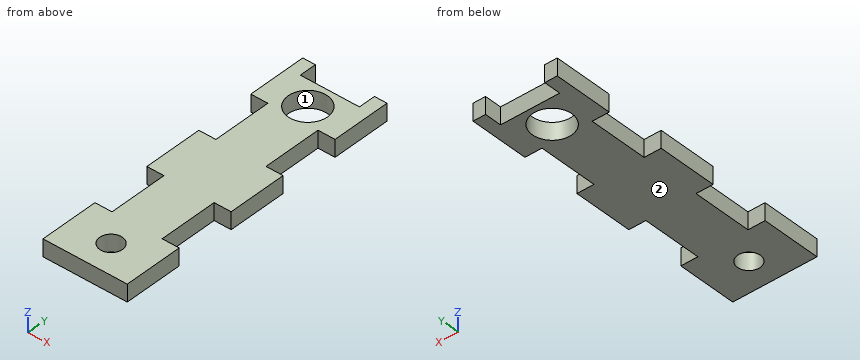
from build123d import *

# Parameters (mm, degrees)
SKETCH1_R               = 11
BOSS_EXTRUDE1_DEPTH     = 9.525
SKETCH3_R               = 6.35
CUT_EXTRUDE1_DEPTH      = 1
CUT_EXTRUDE1_DEPTH_BACK = 10.525


with BuildPart() as part:
    # Sketch1 → Boss-Extrude1 (new body)
    with BuildSketch(Plane.XY):
        Polygon((0, 0), (0, -33.02), (9.525, -33.02), (9.525, -66.04), (0, -66.04), (0, -99.06), (9.525, -99.06), (9.525, -132.08), (0, -132.08), (0, -165.1), (47.05, -165.1), (47.05, -132.08), (37.525, -132.08), (37.525, -99.06), (47.05, -99.06), (47.05, -66.04), (37.525, -66.04), (37.525, -33.02), (47.05, -33.02), (47.05, 0), (40.03499994, 0), (40.03499994, -9.525), (7.01499994, -9.525), (7.01499994, 0), align=None)
        with Locations((23.525, -23.525)):
            Circle(SKETCH1_R, mode=Mode.SUBTRACT)
    extrude(amount=BOSS_EXTRUDE1_DEPTH)

    # Sketch3 → Cut-Extrude1 (cut, two sides)
    with BuildSketch(Plane(origin=(0, 0, 0), x_dir=(-1, 0, 0), z_dir=(0, 0, -1))) as cut_extrude1_sk:
        with Locations((-23.525, -148.59)):
            Circle(SKETCH3_R)
    extrude(amount=CUT_EXTRUDE1_DEPTH, mode=Mode.SUBTRACT)
    extrude(cut_extrude1_sk.sketch, amount=-CUT_EXTRUDE1_DEPTH_BACK, mode=Mode.SUBTRACT)


solid = part.part
Read the model definition and answer for the solid it produces. Units are mm, in the model's axes. Face numbers are marked on the shaded views. Coordinates: 2 decimals unless noted, no trailing zeros. Write each loop counter-clockwise with the first axis right and the second up, starting at its lowest first coordinate (ties: lowest second). Pieces come first, ordered by that corner, then holes. Notation, with made-up numbers: (39.25, 53.5) -> (48.25, 53.5) arc R26 cw to (48.25, 86.5) -> close; hole circle Ø5 at (74.5, -18.5). An arc over 180 degrees is marked (long way). Return JSON: item names as keys, results as strings.
(1) For a pull along X with two mould halves and no side action, classify the marked faces 1 and 2 as pulls with the +X half, pulls with the -X half, needs draft (parallel to the pull), parting line crosses it, or undercut.
Answers below:
{"face 1": "undercut", "face 2": "needs draft"}
(2) The part is cut by section A-A on y = -148.59. Give the vertices of the cut face in (x, z) (3 decimals).
Answers below:
{"outline": "(0, 0) -> (17.175, 0) -> (17.175, 9.525) -> (0, 9.525) -> close; (29.875, 0) -> (47.05, 0) -> (47.05, 9.525) -> (29.875, 9.525) -> close"}
(3) The part is cut by section D-D on y = -30. Give the vertices of the cut face in (x, z) (3 decimals).
Answers below:
{"outline": "(0, 0) -> (14.633, 0) -> (14.633, 9.525) -> (0, 9.525) -> close; (32.417, 0) -> (47.05, 0) -> (47.05, 9.525) -> (32.417, 9.525) -> close"}
(4) Each of these flat-tipped pins is pushed along its axis until it touches: P1, Ø3, axis at y = -44, z = 6.5, coming from the -X side (3 decimals); P2, Ø5, axis at x = 27.5, z = 6, coming from the +Y side (3 decimals); P3, Ø3, axis at y = -108.5, z = 3, coming from the +X side (3 decimals). Where does it stop, or does it pass through?
Answers below:
{"P1": "x = 9.525", "P2": "y = -9.525", "P3": "x = 37.525"}
(5) Consider line 1 along Y through (x, z) = (38, 6.5) (3 decimals); line 2 along Y through (x, z) = (3, 1.75); line 3 along X through (y, z) = (-44, 5) (3 decimals). Determine where each line is inside the solid, lowest interval first. Write a range as from..to.
Answers below:
{"line 1": "-165.1..-132.08, -99.06..-66.04, -33.02..-9.525", "line 2": "-165.1..-132.08, -99.06..-66.04, -33.02..0", "line 3": "9.525..37.525"}
(6) The part is cut by section C-C on x = 22. Give the vertices of the cut face in (y, z) (3 decimals), then the cut area to 3 significant figures.
Answers below:
{"outline": "(-165.1, 0) -> (-154.754, 0) -> (-154.754, 9.525) -> (-165.1, 9.525) -> close; (-142.426, 0) -> (-34.419, 0) -> (-34.419, 9.525) -> (-142.426, 9.525) -> close; (-12.631, 0) -> (-9.525, 0) -> (-9.525, 9.525) -> (-12.631, 9.525) -> close", "area": "1,160 mm^2"}
(7) The part is cut by section B-B on z = 5.5. Give the vertices of the cut face in (x, y) (3 decimals), then the cut area to 3 significant figures.
Answers below:
{"outline": "(0, -165.1) -> (47.05, -165.1) -> (47.05, -132.08) -> (37.525, -132.08) -> (37.525, -99.06) -> (47.05, -99.06) -> (47.05, -66.04) -> (37.525, -66.04) -> (37.525, -33.02) -> (47.05, -33.02) -> (47.05, 0) -> (40.035, 0) -> (40.035, -9.525) -> (7.015, -9.525) -> (7.015, 0) -> (0, 0) -> (0, -33.02) -> (9.525, -33.02) -> (9.525, -66.04) -> (0, -66.04) -> (0, -99.06) -> (9.525, -99.06) -> (9.525, -132.08) -> (0, -132.08) -> close; hole circle Ø22 at (23.525, -23.525); hole circle Ø12.7 at (23.525, -148.59)", "area": "5,690 mm^2"}
